Autodesk Inventor part; units mm, degrees
ref_plane "YZ Plane" through (0, 0, 0) normal (1, 0, 0) x (0, 1, 0)
ref_plane "XZ Plane" through (0, 0, 0) normal (0, 1, 0) x (-1, 0, 0)
ref_plane "XY Plane" through (0, 0, 0) normal (0, 0, 1) x (1, 0, 0)
sketch "스케치1" plane through (0, 0, 0) normal (0, 0, 1) x (1, 0, 0)
  line L0 (16.6105, -9.1135) -> (-16.6105, -9.1135)
  line L1 (-16.6105, -9.1135) -> (-16.6105, 9.1135)
  line L2 (-16.6105, 9.1135) -> (16.6105, 9.1135)
  line L3 (16.6105, 9.1135) -> (16.6105, -9.1135)
  line L4 (16.6105, -9.1135) -> (-16.6105, 9.1135) construction
  line L5 (-16.6105, -9.1135) -> (16.6105, 9.1135) construction
  point P0 (0, 0)
extrude "돌출1" add sketch "스케치1" along normal blind 15
sketch "스케치2" plane through (0, 0, 15) normal (0, 0, 1) x (1, 0, 0)
  line L0 (16.6105, 9.1135) -> (-16.6105, 9.1135)
  line L1 (-8.2042, 9.1135) -> (-12.7307, 0)
  line L2 (-12.7307, 0) -> (8.0426, 0)
  line L3 (8.0426, 0) -> (8.0426, 9.1135)
  point P0 (0, 0)
extrude "돌출2" cut sketch "스케치2" against normal blind 15
sketch "스케치3" plane through (16.6105, -9.1135, 0) normal (1, 0, 0) x (0, 0, -1)
  line L0 (0, 18.2271) -> (-15, 18.2271)
  line L1 (-13.2965, 18.2271) -> (-7.9213, 9.1135)
  line L2 (-15, 9.1135) -> (0, 9.1135)
  line L3 (-7.9213, 9.1135) -> (0, 18.2271)
extrude "돌출3" cut sketch "스케치3" against normal blind 15
properties part number "240503_3Dsketch09"
Check sheet for the modelled part. Datum: model origin and axes. Units: mm. A direction names the side the tool comes from. Give positions to 0.01 mm unless a question says otherwise; leave off trailing zeros. Write each loop counter-clockwise with the first axis right and the second up, starting at its lowest first coordinate (ties: lowest second). Pieces come first, ordered by that corner, then holes.
Item 1: Cross-section at C-C (x = -12). Enter the section's corners in (y, z), and give its area (3 significant figures).
Item 2: Gauge pin test, flat end, axial feed: pin 1 (7.5 mm diameter, centred on x = -7, z = 7, fed in from +Y). Record the tip position at first contact, or that the pin passes through.
Item 3: Access from +Z, -Z, +X, -X, +Y, -Y to the whole of each face (thin tool, end or side, straight path). Record for faces 1 (the face through (8.043, 3, 12)), 2 (the face through (0, -2, 15)), 3 (the face through (-10.436, 4.621, 7.605)), 4 (the face through (12.387, 4.621, 10.646)).
Item 4: Draft check along X on faces 5 (the face through (-16.61, 0, 7)), 6 (the face through (0, -2, 0)), 7 (the face through (-2, 0, 8)). Enter one of: released by +X, released by -X, zero draft, split by the parting line, or undercut.
Item 5: Cross-section at D-D (z = 12.25). Enter the section's corners in (x, y), and give its area (3 significant figures).
Item 6: Scan lines: L1, parallel to Z at x = 14, y = 8.25; L2, parallel to X at y = 3.25, z = 2.5; L3, parallel to Y at x = 2, z = 14.75. Record each from-to range of solid material in increasing order.
Item 7: Cross-section at B-B (y = 6). Enter the section's corners in (x, z).
Report:
1. outline: (-9.11, 0) - (0, 0) - (0, 15) - (-9.11, 15) - close; (1.47, 0) - (9.11, 0) - (9.11, 15) - (1.47, 15) - close
1. area: 251 mm2
2. pin 1: stops at y = 9.11
3. face 1: +Z, -Z, +Y
3. face 2: +Z, +X, -X, +Y, -Y
3. face 3: +Z, -Z
3. face 4: +X, +Y
4. face 5: released by -X
4. face 6: zero draft
4. face 7: undercut
5. outline: (-16.61, -9.11) - (16.61, -9.11) - (16.61, 7.34) - (8.04, 7.34) - (8.04, 0) - (-12.73, 0) - (-8.2, 9.11) - (-16.61, 9.11) - close
5. area: 422 mm2
6. L1: z = 0 to 0.75, 12.79 to 15
6. L2: x = -16.61 to -11.12, 8.04 to 16.61
6. L3: y = -9.11 to 0
7. outline: (-16.61, 0) - (-9.75, 0) - (-9.75, 15) - (-16.61, 15) - close; (8.04, 0) - (16.61, 0) - (16.61, 2.71) - (8.04, 2.71) - close; (8.04, 11.46) - (16.61, 11.46) - (16.61, 15) - (8.04, 15) - close
